The model under review builds one solid part; all positions refer to its coordinate system, in mm. A direction names the side the tool comes from. Coordinates: 2 decimals unless noted, no trailing zeros. Loops run counter-clockwise (first coordinate to the right, second up) from the corner with the lowest first, then second, coordinate; pieces in that order, holes last. Notation, with made-up numbers: (69.5, -25.5) - (111.5, -25.5) arc R14 cw to (111.5, -1.5) - close; hole circle Ø6 at (31, 44.25). An arc over 180 degrees is marked (long way). Use a Markdown table: item, result. Add a question column.
1) Add section B-B, the plane x = -2. Give the boundary of the cut face in (y, z).
2) For faces 5 (the flat face through (0.14, 3.698, 10.14)), 6 (the flat face through (-25, 0, 10)), list the 3-axis set-ups (+Z, -Z, +X, -X, +Y, -Y) from which the entire face can be reached by the end or side of a thin tool; tool diameter is ignored.
3) The part is to be moulded in two halves that separate along Y. For faces 1 (the flat face through (-10, 0, 10)), 2 (the flat face through (0, -15, 10)), 3 (the flat face through (-0.14, -3.802, 10.14)), 4 (the flat face through (0, 15, 10)), say which applies: pulls with the +Y half, pulls with the -Y half, needs draft (parallel to the pull), parting line crosses it, or undercut.
4) Add section C-C, the plane z = 6.75. Give the boundary of the cut face in (x, y).
5) To check wall thickness, follow L1, parallel to Y at x = -6.5, z = 1.5; L2, parallel to Y at x = 3, z = 17.75 (3 decimals). State the ranges of each line that lie inside material, in increasing order. Write a range as [from, to].
6) Add section A-A, the plane y = 1.5. Give the boundary of the cut face in (x, z).
```python
from build123d import *

# Parameters (mm, degrees)
F0_W     = 50
F0_H     = 30
F1_DEPTH = 20
F3_DEPTH = 20.001
F4_R     = 0.5


with BuildPart() as f1:
    # F0 (on Top) → F1 (new body)
    with BuildSketch(Plane.XY):
        Rectangle(F0_W, F0_H)
    extrude(amount=F1_DEPTH)

    # F2 (on face) → F3 (cut, through all)
    with BuildSketch(Plane.XY.offset(20)):
        Polygon((10, 0), (-10, 7.5), (-10, -7.5), align=None)
    extrude(amount=-F3_DEPTH, mode=Mode.SUBTRACT)

    # F4
    f4_edges = [f1.edges().sort_by_distance(p)[0] for p in [
        (-25, -15, 10),
        (25, -15, 10),
        (0, -15, 0),
        (0, -15, 20),
        (-25, 15, 10),
        (-25, 0, 0),
        (-25, 0, 20),
        (25, 15, 10),
        (25, 0, 0),
        (25, 0, 20),
        (0, 15, 0),
        (0, 15, 20),
    ]]
    fillet(f4_edges, radius=F4_R)


solid = f1.part
```
From the geometry:
| question | item | result |
|---|---|---|
| 1 | outline | (-15, 0.5) arc R0.5 ccw to (-14.5, 0) - (-4.5, 0) - (-4.5, 20) - (-14.5, 20) arc R0.5 ccw to (-15, 19.5) - close; (4.5, 0) - (14.5, 0) arc R0.5 ccw to (15, 0.5) - (15, 19.5) arc R0.5 ccw to (14.5, 20) - (4.5, 20) - close |
| 2 | face 5 | +Z, -Z |
| 2 | face 6 | +Z, -Z, -X, +Y, -Y |
| 3 | face 1 | undercut |
| 3 | face 2 | pulls with the -Y half |
| 3 | face 3 | undercut |
| 3 | face 4 | pulls with the +Y half |
| 4 | outline | (-25, -14.5) arc R0.5 ccw to (-24.5, -15) - (24.5, -15) arc R0.5 ccw to (25, -14.5) - (25, 14.5) arc R0.5 ccw to (24.5, 15) - (-24.5, 15) arc R0.5 ccw to (-25, 14.5) - close; hole (-10, -7.5) - (10, 0) - (-10, 7.5) - close |
| 5 | L1 | y = [-15, -6.19], [6.19, 15] |
| 5 | L2 | y = [-15, -2.625], [2.625, 15] |
| 6 | outline | (-25, 0.5) arc R0.5 ccw to (-24.5, 0) - (-10, 0) - (-10, 20) - (-24.5, 20) arc R0.5 ccw to (-25, 19.5) - close; (6, 0) - (24.5, 0) arc R0.5 ccw to (25, 0.5) - (25, 19.5) arc R0.5 ccw to (24.5, 20) - (6, 20) - close |
